Input: dimensioned drawing with shaded views. Units: mm. Origin: part minimum x, y, z. A direction names the side the tool comes from. Give positions to 0.01 mm unless a question says otherwise; leave off trailing zeros. Write each loop counter-clockwise with the first axis right and the second up, starting at its lowest first coordinate (ties: lowest second). Pieces come first, ordered by that corner, then holes.
Q1. Mould query, pull axis Z, two halves, no side actions, for the marked faces 1, 2 and 3. Classes: +Z half, -Z half, draft (parallel to the pull), parting line (faces both ways), or undercut.
Q2. Line query: line 1 (X direction, y = 1, z = 20); line 2 (Y direction, x = 41, z = 20); line 3 (Y direction, x = 34.5, z = 18). Output: solid intervals per line, ascending.
Q3. Section D-D (x = 42). Return the cut outline in (y, z), plus the area to 3 significant figures.
Q4. Section C-C (z = 20). Return the cut outline in (x, y), plus the area to 3 significant figures.
Q5. Section A-A (x = 20). Return the cut outline in (y, z), plus the area to 3 significant figures.
Q6. Reachability of the marked faces 4 and 5 from +Z, -Z, +X, -X, +Y, -Y: full face, straight path, thin tool, end or side. Return the list, or none.
Q7. Section B-B (y = 20). Return the cut outline in (x, z).
Q8. Pin query (flat end, axial travel): pin 1 Ø10 at (x, z) = (30, 11.5) entering from +Y; pin 2 Ø10.5 at (y, z) = (17, 21) entering from -X. Return the tip coordinate at first contact, or that it passes through.
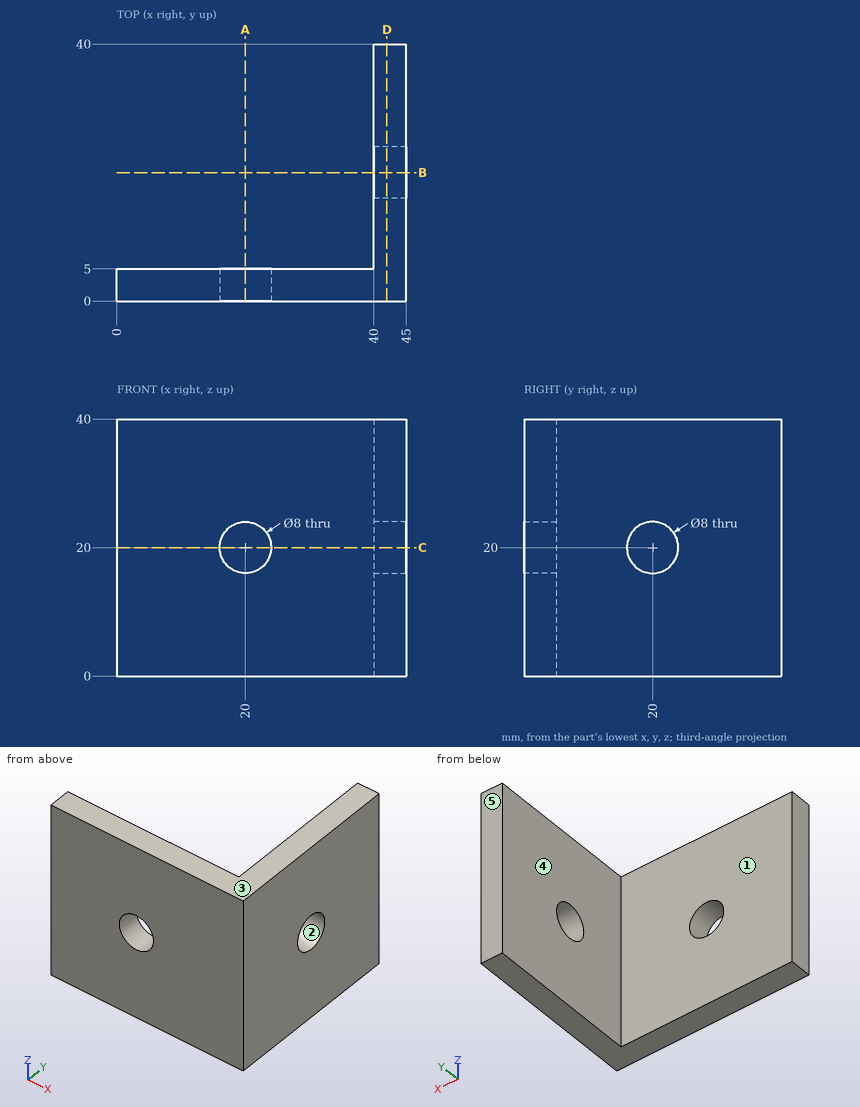
Computed:
1. face 1: draft
1. face 2: undercut
1. face 3: +Z half
2. line 1: x = 0 to 16, 24 to 45
2. line 2: y = 0 to 16, 24 to 40
2. line 3: y = 0 to 5
3. outline: (0, 0) - (40, 0) - (40, 40) - (0, 40) - close; hole circle Ø8 at (20, 20)
3. area: 1,550 mm2
4. outline: (0, 0) - (16, 0) - (16, 5) - (0, 5) - close; (24, 0) - (45, 0) - (45, 16) - (40, 16) - (40, 5) - (24, 5) - close; (40, 24) - (45, 24) - (45, 40) - (40, 40) - close
4. area: 320 mm2
5. outline: (0, 0) - (5, 0) - (5, 16) - (0, 16) - close; (0, 24) - (5, 24) - (5, 40) - (0, 40) - close
5. area: 160 mm2
6. face 4: +Z, -Z, -X, +Y
6. face 5: +Z, -Z, +X, -X, +Y
7. outline: (40, 0) - (45, 0) - (45, 16) - (40, 16) - close; (40, 24) - (45, 24) - (45, 40) - (40, 40) - close
8. pin 1: stops at y = 5
8. pin 2: stops at x = 40
